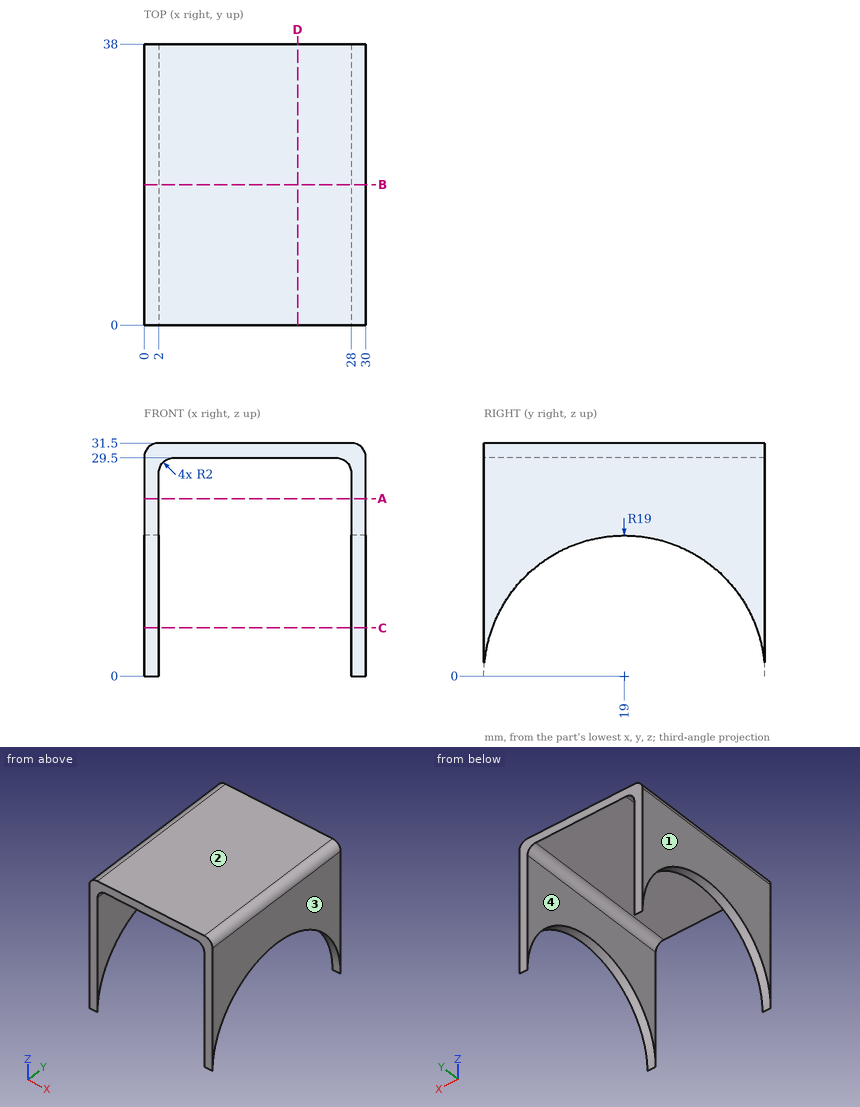
Source: three-view drawing plus pictorial views. Frame: mm from the lowest corner of the part. Coordinates: 2 decimals unless noted, no trailing zeros. Write each loop counter-clockwise with the first axis right and the second up, starting at its lowest first coordinate (ties: lowest second). Pieces come first, ordered by that corner, then holes. Notation, with made-up numbers: (20.5, 51.5) -> (79.5, 51.5) arc R19 ccw to (79.5, 67.5) -> close; hole circle Ø7 at (-15.5, 31). An arc over 180 degrees is marked (long way). Answer as a JSON object with one key per item and string values.
1. Section D-D on x = 20.75. Return the cut outline in (y, z), then the cut area to 3 significant figures.
Result set:
{"outline": "(0, 29.5) -> (38, 29.5) -> (38, 31.5) -> (0, 31.5) -> close", "area": "76.0 mm2"}
2. Section B-B on y = 19. Return the cut outline in (x, z), then the cut area to 3 significant figures.
Result set:
{"outline": "(0, 19) -> (2, 19) -> (2, 27.5) arc R2 cw to (4, 29.5) -> (26, 29.5) arc R2 cw to (28, 27.5) -> (28, 19) -> (30, 19) -> (30, 29.5) arc R2 ccw to (28, 31.5) -> (2, 31.5) arc R2 ccw to (0, 29.5) -> close", "area": "102 mm2"}
3. Mould query, pull axis X, two halves, no side actions, for the marked faces 1, 2, 3 and 4. Classes: released by +X, released by -X, zero draft, split by the parting line, or undercut.
Result set:
{"face 1": "released by -X", "face 2": "zero draft", "face 3": "released by +X", "face 4": "undercut"}
4. First-contact query: P1, Ø8, axis at y = 22.5, z = 24.5, coming from the -X side; P2, Ø12, axis at y = 11.5, z = 9, coming from the -X side; P3, Ø12, axis at x = 9.5, y = 14.5, coming from the -Z side. Flat tips, straight axial feed; report the tip coordinate or a pass-through.
Result set:
{"P1": "stops at x = 0", "P2": "passes through", "P3": "stops at z = 29.44"}
5. Material intervals for line 1 (X direction, y = 21, z = 27); line 2 (Z direction, x = 12.75, y = 35); line 3 (Z direction, x = 28.25, y = 35), sorted ascending. Write a range as from..to.
Result set:
{"line 1": "x = 0..2, 28..30", "line 2": "z = 29.5..31.5", "line 3": "z = 10.25..31.48"}
6. Section A-A on z = 24. Return the cut outline in (x, y), then the cut area to 3 significant figures.
Result set:
{"outline": "(0, 0) -> (2, 0) -> (2, 38) -> (0, 38) -> close; (28, 0) -> (30, 0) -> (30, 38) -> (28, 38) -> close", "area": "152 mm2"}
7. Section C-C on z = 6.5. Return the cut outline in (x, y), then the cut area to 3 significant figures.
Result set:
{"outline": "(0, 0) -> (2, 0) -> (2, 1.15) -> (0, 1.15) -> close; (0, 36.85) -> (2, 36.85) -> (2, 38) -> (0, 38) -> close; (28, 0) -> (30, 0) -> (30, 1.15) -> (28, 1.15) -> close; (28, 36.85) -> (30, 36.85) -> (30, 38) -> (28, 38) -> close", "area": "9.17 mm2"}
